The listing builds one solid part. Answer for the finished solid, in the listing's coordinates (mm). A direction names the side the tool comes from. Coordinates: 2 decimals unless noted, no trailing zeros. Order: outer loops, then holes, each group sorted by start corner. A loop starts at its lowest first (then second) coordinate and runs counter-clockwise, first axis right, second up. Notation, with made-up numbers: (34.5, -1.75) - (85.5, -1.75) arc R29 cw to (85.5, 30.25) - close; hole circle Ø2 at (-17, -6). An arc over 180 degrees is marked (long way). One line per item, written item: value. Start each with the question number.
```python
from build123d import *

# Parameters (mm, degrees)
BOSS_EXTRUDE1_DEPTH      = 355.6
BOSS_EXTRUDE1_DEPTH_BACK = 355.6
SKETCH1_W                = 50.8
SKETCH1_H                = 50.8
SKETCH1_W_2              = 44.45
SKETCH1_H_2              = 44.45
SKETCH2_R                = 14.2875
CUT_EXTRUDE1_DEPTH       = 361.10715072
FILLET1_R                = 3.175


with BuildPart() as part:
    # Sketch1 → Boss-Extrude1 (new, two sides: drawn at the far end of the back side and taken through both)
    with BuildSketch(Plane.XY.offset(-BOSS_EXTRUDE1_DEPTH_BACK)):
        Rectangle(SKETCH1_W, SKETCH1_H)
        Rectangle(SKETCH1_W_2, SKETCH1_H_2, mode=Mode.SUBTRACT)
    extrude(amount=BOSS_EXTRUDE1_DEPTH + BOSS_EXTRUDE1_DEPTH_BACK)

    # Sketch2 → Cut-Extrude1 (cut, through all)
    with BuildSketch(Plane.ZY.offset(25.4)):
        with Locations((-295.240391678, 1.5875)):
            Circle(SKETCH2_R)
        Circle(SKETCH2_R)
        with Locations((295.240391678, 1.5875)):
            Circle(SKETCH2_R)
    extrude(amount=-CUT_EXTRUDE1_DEPTH, mode=Mode.SUBTRACT)

    # Fillet1
    fillet1_edges = [part.edges().sort_by_distance(p)[0] for p in [
        (0, -25.4, -355.6),
        (0, 25.4, 355.6),
        (0, -25.4, 355.6),
        (0, 25.4, -355.6),
    ]]
    fillet(fillet1_edges, radius=FILLET1_R - 0.0001)  # a hair under: the kernel refuses the full size


solid = part.part
```
(1) The part is cut by section B-B on z = 0. Determine the outline of the cut face in (x, y) (1 decimal).
(2) Consider probe 1 along Y at (x, z) = (11, 99) (3 decimals); probe 2 along Y at (x, z) = (-23.4, 0). Determine where each line is inside the solid, lowest interval first.
(3) For a pull along Y with two mould halves and no side action, classify faces 3 (the face through (-23, 0, 355.6)), 4 (the face through (0, 25.4, -5)), 5 (the face through (0, -25.4, -5)), 6 (the face through (0, 22.225, -5)) as pulls with the +Y half, pulls with the -Y half, needs draft (parallel to the pull), parting line crosses it, or undercut.
(4) Flat-ended cylindrical pins translate along their axes: pin 1 Ø23 at (y, z) = (0, 0) entering from -X; pin 2 Ø10 at (x, y) = (-1.5, 17.5) entering from -Z. Find the tip coordinate at first contact, or state that the pin passes through.
(5) For faces 1 (the face through (-22.225, -15, -5)), 2 (the face through (-23.835, 0.628, -14.274)), determine the directions among +Z, -Z, +X, -X, +Y, -Y from which every point of the face is accessible in a straight line to the end or side of a thin tool.
Completed:
1. outline: (-25.4, -25.4) - (25.4, -25.4) - (25.4, -14.3) - (22.2, -14.3) - (22.2, -22.2) - (-22.2, -22.2) - (-22.2, -14.3) - (-25.4, -14.3) - close; (-25.4, 14.3) - (-22.2, 14.3) - (-22.2, 22.2) - (22.2, 22.2) - (22.2, 14.3) - (25.4, 14.3) - (25.4, 25.4) - (-25.4, 25.4) - close
2. probe 1: y = -25.4 to -22.225, 22.225 to 25.4
2. probe 2: y = -25.4 to -14.29, 14.29 to 25.4
3. face 3: needs draft
3. face 4: pulls with the +Y half
3. face 5: pulls with the -Y half
3. face 6: undercut
4. pin 1: passes through
4. pin 2: stops at z = -355.6
5. face 1: +Z, -Z
5. face 2: +X, -X
